Here's how the part is built. I have some questions about the finished solid (model axes, mm). A direction names the side the tool comes from. Round coordinates to 2 decimals unless told otherwise and drop trailing zeros. Loops run counter-clockwise (first coordinate to the right, second up) from the corner with the lowest first, then second, coordinate; pieces in that order, holes last. Notation, with made-up numbers: (63.25, -7) -> (80.25, -7) arc R22 ccw to (80.25, 5) -> close; hole circle Ø11 at (2, -20.5). An arc over 180 degrees is marked (long way). One line per item, written item: value. Start each with the question number.
```python
from build123d import *

# Parameters (mm, degrees)
BOSS_EXTRUDE1_DEPTH = 40
SKETCH4_W           = 11.8
SKETCH4_H           = 32.3
CUT_EXTRUDE1_DEPTH  = 5.5
SKETCH5_W           = 11.8
SKETCH5_H           = 22.5
CUT_EXTRUDE2_DEPTH  = 9.498848241
SKETCH6_R           = 1.25
CUT_EXTRUDE3_DEPTH  = 9.498848241
BOSS_EXTRUDE2_DEPTH = 12
SKETCH8_W           = 8
SKETCH8_H           = 10
CUT_EXTRUDE4_DEPTH  = 10
SKETCH9_R           = 2
CUT_EXTRUDE5_DEPTH  = 30.384991323


with BuildPart() as part:
    # Sketch1 → Boss-Extrude1 (new body)
    with BuildSketch(Plane.XY):
        Polygon((8.670952565, 9.003587153), (-11.329047435, 9.003587153), (-21.329047435, 9.003587153), (-21.329047435, -4.995261088), (-11.329047435, -4.995261088), (8.670952565, -4.995261088), align=None)
    extrude(amount=BOSS_EXTRUDE1_DEPTH)

    # Sketch4 → Cut-Extrude1 (cut)
    with BuildSketch(Plane(origin=(0, 9.003587153, 0), x_dir=(1, 0, 0), z_dir=(0, 1, 0))):
        with Locations((-6.329047435, -20)):
            Rectangle(SKETCH4_W, SKETCH4_H)
    extrude(amount=-CUT_EXTRUDE1_DEPTH, mode=Mode.SUBTRACT)

    # Sketch5 → Cut-Extrude2 (cut, through all)
    with BuildSketch(Plane(origin=(0, 3.503587153, 0), x_dir=(1, 0, 0), z_dir=(0, 1, 0))):
        with Locations((-6.329047435, -20)):
            Rectangle(SKETCH5_W, SKETCH5_H)
    extrude(amount=-CUT_EXTRUDE2_DEPTH, mode=Mode.SUBTRACT)

    # Sketch6 → Cut-Extrude3 (cut, through all)
    with BuildSketch(Plane(origin=(0, 3.503587153, 0), x_dir=(1, 0, 0), z_dir=(0, 1, 0))):
        with Locations((-6.329047435, -6.3)):
            Circle(SKETCH6_R)
        with Locations((-6.329047435, -33.7)):
            Circle(SKETCH6_R)
    extrude(amount=-CUT_EXTRUDE3_DEPTH, mode=Mode.SUBTRACT)

    # Sketch7 → Boss-Extrude2 (add)
    with BuildSketch(Plane.XY):
        Polygon((8.670952565, 9.003587153), (8.670952565, -4.995261088), (11.458506302, -4.995261088), (24.231440373, 0.295461436), (20.787289482, 8.610377228), (18.87387232, 13.229774891), align=None)
    extrude(amount=BOSS_EXTRUDE2_DEPTH)

    # Sketch8 → Cut-Extrude4 (cut)
    with BuildSketch(Plane(origin=(20.787289482, 8.610377228, 0), x_dir=(0, 0, -1), z_dir=(0.923879533, 0.382683432, 0))):
        with Locations((-6, -2)):
            Rectangle(SKETCH8_W, SKETCH8_H)
    extrude(amount=-CUT_EXTRUDE4_DEPTH, mode=Mode.SUBTRACT)

    # Sketch9 → Cut-Extrude5 (cut, through all)
    with BuildSketch(Plane(origin=(3.444150891, -8.314915793, 0), x_dir=(0.923879533, 0.382683432, 0), z_dir=(0.382683432, -0.923879533, 0))):
        with Locations((15.587337893, 6)):
            Circle(SKETCH9_R)
    extrude(amount=-CUT_EXTRUDE5_DEPTH, mode=Mode.SUBTRACT)


solid = part.part
```
Q1. I want a section at C-C on y = 1.5. Please give me the cut outline in (x, z).
Q2. Which directions (+Z, -Z, +X, -X, +Y, -Y) give clear straight access to the entire face, cutting with the end or side of a thin tool? Please do faces 1 (the flat face through (-6, -1, 31.25)), 2 (the flat face through (15, 4, 12)), 3 (the flat face through (-8, 3.504, 34)), 4 (the flat face through (1, 9.004, 20)), 5 (the flat face through (17, 5, 2)).
Q3. Will these pins go through, and if not, where does the flat tip stop? P1, Ø1.5, axis at x = -6.33, z = 6.3, coming from the -Y side; P2, Ø8, axis at x = 19, y = 2.5, coming from the +Z side; P3, Ø15, axis at x = -7.5, z = 20, coming from the +Y side; P4, Ø5.5, axis at x = -8, z = 7.5, coming from the +Y side.
Q4. If I drill on line 1 along X through (y, z) = (-3.25, 19); line 2 along X through (y, z) = (1, 33.7); line 3 along Z through (x, y) = (18.5, 7), over which ranges is the centre line in solid material (lowest first)?
Q5. If we mould it in two halves opening along X, with no side actions, what happens to faces 6 (the flat face through (1, 2, 0)), 7 (the flat face through (16.336, -2.975, 4.583)), 8 (the cylindrical face through (11.514, 9.083, 7.352))? For each: released by +X, released by -X, zero draft, split by the parting line, or undercut.
Q6. I want a section at B-B on z = 16. Please give me the cut outline in (x, y), plus the area to 3 significant figures.
Q7. I want a section at A-A on z = 33.7. Please give me the cut outline in (x, y).
Answers below:
1. outline: (-21.33, 0) -> (23.73, 0) -> (23.73, 12) -> (8.67, 12) -> (8.67, 40) -> (-21.33, 40) -> close; hole (-12.23, 8.75) -> (-0.43, 8.75) -> (-0.43, 31.25) -> (-12.23, 31.25) -> close; hole circle Ø2.5 at (-6.33, 6.3); hole circle Ø2.5 at (-6.33, 33.7); hole (12.91, 2) -> (21.91, 2) -> (21.91, 10) -> (12.91, 10) -> close
2. face 1: +Y, -Y
2. face 2: +Z, +X, +Y, -Y
2. face 3: +Y
2. face 4: +Z, -Z, -X, +Y
2. face 5: none
3. P1: passes through
3. P2: stops at z = 12
3. P3: stops at y = 9
3. P4: stops at y = 3.5
4. line 1: x = -21.33 to -12.23, -0.43 to 8.67
4. line 2: x = -21.33 to -7.58, -5.08 to 8.67
4. line 3: z = 0 to 2, 10 to 12
5. face 6: zero draft
5. face 7: released by +X
5. face 8: undercut
6. outline: (-21.33, -5) -> (-12.23, -5) -> (-12.23, 9) -> (-21.33, 9) -> close; (-0.43, -5) -> (8.67, -5) -> (8.67, 9) -> (-0.43, 9) -> close
6. area: 255 mm^2
7. outline: (-21.33, -5) -> (-7.58, -5) -> (-7.58, 3.5) -> (-12.23, 3.5) -> (-12.23, 9) -> (-21.33, 9) -> close; (-5.08, -5) -> (8.67, -5) -> (8.67, 9) -> (-0.43, 9) -> (-0.43, 3.5) -> (-5.08, 3.5) -> close
